Here's how the part is built. I have some questions about the finished solid (model axes, mm). A direction names the side the tool comes from. Give positions to 0.01 mm unless a question says otherwise; leave off trailing zeros. Write each loop counter-clockwise with the first axis right and the second up, starting at its lowest first coordinate (ties: lowest second). Pieces come first, ordered by that corner, then holes. Notation, with made-up numbers: M 28,70 L 39,70 A26 ccw 39,90 Z; hole C -9,-33 d1. An arc over 180 degrees is marked long. Answer as CSV lines item,"result". Start each with the question number.
Q1. On a 3-axis mill with a long thin cutter (end or side, diameter ignored), from which of +Z, -Z, +X, -X, +Y, -Y can I reach the whole of each face in a straight line? I mean faces 5 (the cylindrical face through (54.728, 21.025, 2.535)), 6 (the flat face through (15, 25, 2)), 7 (the cylindrical face through (49.032, 26.324, 4.507)). Say none if no direction works.
Q2. Thinking about a two-plate mould opening in Y: for faces 1 (the flat face through (44, 12, 0)), 2 (the flat face through (39, 23, 4)), 3 (the flat face through (44, 0, 2)), 4 (the cylindrical face through (3.784, 21.115, 2.535)), which applies, +Y half, -Y half, draft (parallel to the pull), parting line (faces both ways), or undercut?
Q3. Suppose I cut it at A-A (x = 45). Write out the boundary of the cut face in (y, z).
Q4. Suppose I cut it at D-D (y = 14.5). Write out the boundary of the cut face in (x, z).
Q5. For pin 1 (2.5 mm diameter, centred on x = 65, y = 20, fed in from -Z); pin 2 (1 mm diameter, centred on x = 9, z = 0.5, fed in from +Y); pin 3 (4.5 mm diameter, centred on x = 41.5, y = 17.5, fed in from +Z), each with a flat end and sliding along its axis, tell me the tip position at first contact or that it passes through.
Q6. Suppose I cut it at C-C (x = 85). Write out the boundary of the cut face in (y, z), then the cut area to 3 significant figures.
Q7. Suppose I cut it at B-B (z = 1.6). Count the separate pieces of the cut face and the enclosed holes in it, then the cut area to 3 significant figures.
Q8. If I drill on line 1 along Y through (x, z) = (85, 1.1); line 2 along Y through (x, z) = (45.5, 4.3); line 3 along X through (y, z) = (6.25, 1.85), over which ranges is the centre line in solid material (lowest first)?
```python
from build123d import *

# Parameters (mm, degrees)
ESQUISSE1_W             = 90
ESQUISSE1_H             = 25
BOSS_EXTRU_1_DEPTH      = 5
ESQUISSE6_W             = 20
ESQUISSE6_H             = 5
BOSS_EXTRU_2_DEPTH      = 5
ESQUISSE3_R             = 6.5
ENL_V_MAT_EXTRU_2_DEPTH = 96
ESQUISSE4_R             = 1.05
ENL_V_MAT_EXTRU_3_DEPTH = 96
ESQUISSE5_R             = 1.65
ENL_V_MAT_EXTRU_4_DEPTH = 5
CHANFREIN1_SIZE         = 5
ESQUISSE7_R             = 7.5
ENL_V_MAT_EXTRU_5_DEPTH = 1


with BuildPart() as part:
    # Esquisse1 → Boss.-Extru.1 (new body)
    with BuildSketch(Plane.XY):
        with Locations((45, 12.5)):
            Rectangle(ESQUISSE1_W, ESQUISSE1_H)
    extrude(amount=BOSS_EXTRU_1_DEPTH)

    # Esquisse6 → Boss.-Extru.2 (add)
    with BuildSketch(Plane.XY.offset(5)):
        with Locations((45, 27.5)):
            Rectangle(ESQUISSE6_W, ESQUISSE6_H)
    extrude(amount=-BOSS_EXTRU_2_DEPTH)

    # Esquisse3 → Enlèv. mat.-Extru.2 (cut, through all)
    with BuildSketch(Plane.XY.offset(5)):
        with Locations((45, 20)):
            Circle(ESQUISSE3_R)
    extrude(amount=-ENL_V_MAT_EXTRU_2_DEPTH, mode=Mode.SUBTRACT)

    # Esquisse4 → Enlèv. mat.-Extru.3 (cut, through all)
    with BuildSketch(Plane.XY.offset(5)):
        with Locations((34.5, 4.25)):
            Circle(ESQUISSE4_R)
        with Locations(Location((54.5, 20, 0), (0, 0, 180))):
            Circle(ESQUISSE4_R)
        with Locations(Location((55.5, 4.25, 0), (0, 0, 180))):
            Circle(ESQUISSE4_R)
        with Locations((35.5, 20)):
            Circle(ESQUISSE4_R)
    extrude(amount=-ENL_V_MAT_EXTRU_3_DEPTH, mode=Mode.SUBTRACT)

    # Esquisse5 → Enlèv. mat.-Extru.4 (cut)
    with BuildSketch(Plane.XY.offset(5)):
        with Locations((5, 20)):
            Circle(ESQUISSE5_R)
        with Locations((25, 20)):
            Circle(ESQUISSE5_R)
        with Locations(Location((25, 5, 0), (0, 0, 180))):
            Circle(ESQUISSE5_R)
        with Locations(Location((5, 5, 0), (0, 0, 180))):
            Circle(ESQUISSE5_R)
        with Locations((85, 5)):
            Circle(ESQUISSE5_R)
        with Locations((65, 5)):
            Circle(ESQUISSE5_R)
        with Locations(Location((65, 20, 0), (0, 0, 180))):
            Circle(ESQUISSE5_R)
        with Locations(Location((85, 20, 0), (0, 0, 180))):
            Circle(ESQUISSE5_R)
    extrude(amount=-ENL_V_MAT_EXTRU_4_DEPTH, mode=Mode.SUBTRACT)

    # Chanfrein1
    chanfrein1_edges = [part.edges().sort_by_distance(p)[0] for p in [
        (55, 25, 2.5),
        (35, 25, 2.5),
    ]]
    chamfer(chanfrein1_edges, length=CHANFREIN1_SIZE - 0.0001)  # a hair under: the kernel refuses the full size

    # Esquisse7 → Enlèv. mat.-Extru.5 (cut)
    with BuildSketch(Plane.XY.offset(5)):
        with Locations((45, 20)):
            Circle(ESQUISSE7_R)
    extrude(amount=-ENL_V_MAT_EXTRU_5_DEPTH, mode=Mode.SUBTRACT)


solid = part.part
```
Resolved:
1,face 5,"+Z, -Z"
1,face 6,"+Z, -Z, -X, +Y"
1,face 7,"+Z"
2,face 1,"draft"
2,face 2,"undercut"
2,face 3,"-Y half"
2,face 4,"undercut"
3,outline,"M 0,0 L 13.5,0 L 13.5,4 L 12.5,4 L 12.5,5 L 0,5 Z; M 26.5,0 L 30,0 L 30,5 L 27.5,5 L 27.5,4 L 26.5,4 Z"
4,outline,"M 0,0 L 41.54,0 L 41.54,4 L 39.9,4 L 39.9,5 L 0,5 Z; M 48.46,0 L 90,0 L 90,5 L 50.1,5 L 50.1,4 L 48.46,4 Z"
5,pin 1,"through"
5,pin 2,"y = 25"
5,pin 3,"z = 4"
6,outline,"M 0,0 L 3.35,0 L 3.35,5 L 0,5 Z; M 6.65,0 L 18.35,0 L 18.35,5 L 6.65,5 Z; M 21.65,0 L 25,0 L 25,5 L 21.65,5 Z"
6,area,"92.0 mm^2"
7,separate pieces,"1"
7,enclosed holes,"13"
7,area,"2,160 mm^2"
8,line 1,"0 to 3.35, 6.65 to 18.35, 21.65 to 25"
8,line 2,"0 to 12.52, 27.48 to 30"
8,line 3,"0 to 3.92, 6.08 to 23.92, 26.08 to 63.92, 66.08 to 83.92, 86.08 to 90"
